For this review, take the finished solid that the model builds, in its own axes (mm). Face numbers are marked on the shaded views. A direction names the side the tool comes from. Coordinates: 2 decimals unless noted, no trailing zeros. Order: outer loops, then holes, each group sorted by start corner. A loop starts at its lowest first (then second) coordinate and runs counter-clockwise, first axis right, second up. Notation, with made-up numbers: (85.25, 59) -> (102.25, 59) arc R35 cw to (102.25, 95) -> close; hole circle Ø11 at (-7, 18). An arc over 180 degrees is marked (long way). Return JSON: item names as keys, results as strings. Group by question number.
Item 1: Draft analysis for pull direction Y (two halves, no side actions). For the marked faces 4, 5 and 6, state which applies: +Y half, -Y half, draft (parallel to the pull), parting line (faces both ways), or undercut.
Item 2: Take a section at C-C (y = 0.5). Write out the cut boundary in (x, z).
Item 3: Insertion check: pin 1 (6 mm diameter, centred on x = 0.5, z = -6, fed in from +Y); pin 2 (1.5 mm diameter, centred on y = -9, z = -6, fed in from +X); pin 3 (3 mm diameter, centred on y = 13.5, z = -7.5, fed in from -X). Each pin has a flat end and moves straight along its axis. Give the tip position at first contact, or say it passes through.
Item 4: Take a section at A-A (x = 0). Write out the cut boundary in (y, z).
Item 5: Machinability: for the marked faces 1, 2 and 3, which of the approach directions +Z, -Z, +X, -X, +Y, -Y give a long, thin tool a straight path to every point of the face, cutting with its end or side? Answer none if there is none.
Item 6: Take a section at D-D (z = -8.5). Write out the cut boundary in (x, y).
Item 7: For line 1 along Y through (x, z) = (0, -3); line 2 along Z through (x, y) = (-7, -14); line 3 along X through (y, z) = (3.5, -5.5), list the stretches that pass through material, from the lowest coordinate up.
Item 8: Take a section at B-B (z = -4.5). Write out the cut boundary in (x, y), then the cut area to 3 significant figures.
Autodesk Inventor part; units mm, degrees
ref_plane "YZ Plane" through (0, 0, 0) normal (1, 0, 0) x (0, 1, 0)
ref_plane "XZ Plane" through (0, 0, 0) normal (0, 1, 0) x (-1, 0, 0)
ref_plane "XY Plane" through (0, 0, 0) normal (0, 0, 1) x (1, 0, 0)
sketch "Sketch1" plane through (0, 0, 0) normal (0, 0, 1) x (1, 0, 0)
  line L0 (3.6662, 6.35) -> (7.3323, 0)
  line L1 (7.3323, 0) -> (3.6662, -6.35)
  line L2 (3.6662, -6.35) -> (-3.6662, -6.35)
  line L3 (-3.6662, -6.35) -> (-7.3323, 0)
  line L4 (-7.3323, 0) -> (-3.6662, 6.35)
  line L5 (-3.6662, 6.35) -> (3.6662, 6.35)
  circle A0 centre (0, 0) radius 12.7
  circle A1 centre (0, 0) radius 7.3323 construction
  dimension "d0" = 12.7
  dimension "d2" = 25.4
  dimension "d3" = 5.3677
extrude "Extrusion1" add sketch "Sketch1" against normal blind 6.35
sketch "Sketch2" plane through (0, 0, -6.35) normal (0, 0, -1) x (-1, 0, 0)
  line L0 (7.3323, 0) -> (3.6662, -6.35)
  line L1 (3.6662, -6.35) -> (-3.6662, -6.35)
  line L2 (-3.6662, -6.35) -> (-7.3323, 0)
  line L3 (-7.3323, 0) -> (-3.6662, 6.35)
  line L4 (-3.6662, 6.35) -> (3.6662, 6.35)
  line L5 (3.6662, 6.35) -> (7.3323, 0)
  line L6 (7.3323, 0) -> (3.6662, -6.35)
  line L7 (-10.9985, 19.05) -> (10.9985, 19.05)
  line L8 (10.9985, 19.05) -> (21.997, 0)
  line L9 (21.997, 0) -> (10.9985, -19.05)
  line L10 (10.9985, -19.05) -> (-10.9985, -19.05)
  line L11 (-10.9985, -19.05) -> (-21.997, 0)
  line L12 (-21.997, 0) -> (-10.9985, 19.05)
  point P0 (0, 0)
  point P1 (0, 0)
  point P2 (0, 0)
  dimension "d7" = 12.7
  dimension "d10" = 38.1
extrude "Extrusion3" add sketch "Sketch2" along normal blind 6.35
thicken "Thicken Internal Hex Hold" operation add thickness 0.127 both sides no extend neighbours yes toward (0, 1, 0) faces at (1.2221, 6.35, -8.4667) (-4.8882, 4.2333, -8.4667) (1.2221, 14.8167, -12.7) (6.1103, -2.1167, -8.4667) (1.2221, -6.35, -8.4667) (-4.8882, -4.2333, -4.2333)
thicken "Reduce Size of Bushing Fitting" operation add thickness 0.127 both sides no extend neighbours yes toward (-0.9967573, 0.0804666, 0) faces at (12.6588, -1.0219, -4.2333)
equation "\"d13\" = printSpacing"
equation "\"d14\" = printSpacing"
equation "\"d15\" = printSpacing"
equation "\"d16\" = printSpacing"
equation "\"hexSize\" = 12.7"
equation "\"printSpacing\" = 0.127"
properties part number "1_2x1-hexBushing" material "PC/ABS Plastic"
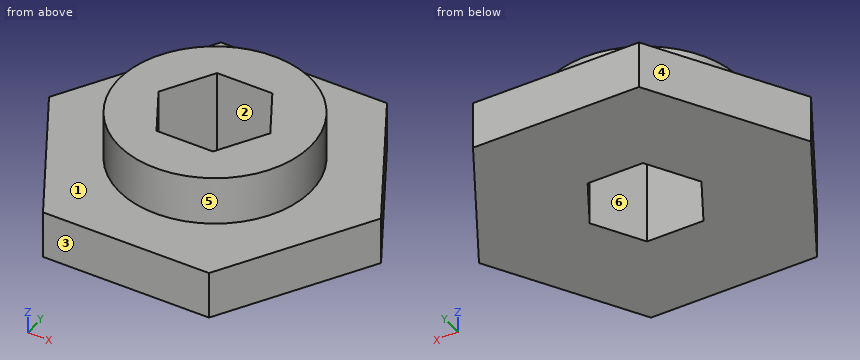
Findings below:
{
 "1": {"face 4": "+Y half", "face 5": "parting line", "face 6": "undercut"},
 "2": {"outline": "(-21.71, -12.57) -> (-7.19, -12.57) -> (-7.19, 0) -> (-12.56, 0) -> (-12.56, -6.35) -> (-21.71, -6.35) -> close; (7.04, -12.57) -> (21.71, -12.57) -> (21.71, -6.35) -> (12.56, -6.35) -> (12.56, 0) -> (7.04, 0) -> close"},
 "3": {"pin 1": "stops at y = 19.05", "pin 2": "stops at x = 17.18", "pin 3": "stops at x = -15.07"},
 "4": {"outline": "(-19.05, -12.57) -> (-6.48, -12.57) -> (-6.48, 0) -> (-12.57, 0) -> (-12.57, -6.35) -> (-19.05, -6.35) -> close; (6.48, -12.57) -> (19.05, -12.57) -> (19.05, -6.35) -> (12.57, -6.35) -> (12.57, 0) -> (6.48, 0) -> close"},
 "5": {"face 1": "+Z", "face 2": "+Z, -Z", "face 3": "+Z, -Z, +X, -X, -Y"},
 "6": {"outline": "(-22, 0) -> (-11, -19.05) -> (11, -19.05) -> (22, 0) -> (11, 19.05) -> (-11, 19.05) -> close; hole (-7.48, 0) -> (-3.74, -6.48) -> (3.74, -6.48) -> (7.41, -0.13) -> (3.59, 6.48) -> (-3.74, 6.48) -> close"},
 "7": {"line 1": "y = -12.57 to -6.48, 6.48 to 12.57", "line 2": "z = -12.57 to -6.35", "line 3": "x = -12.08 to -5.46, 5.31 to 12.08"},
 "8": {"outline": "circle Ø25.15 at (0, 0); hole (-7.48, 0) -> (-3.74, -6.48) -> (3.74, -6.48) -> (7.41, -0.13) -> (3.59, 6.48) -> (-3.74, 6.48) -> close", "area": "352 mm2"}
}
